from build123d import *
from build123d.topology import SkipClean

# Parameters (mm, degrees)
IZIM1_R                     = 6.5
Y_KSEKLIK_EKSTR_ZYON2_DEPTH = 15
IZIM2_R                     = 30
Y_KSEKLIK_EKSTR_ZYON3_DEPTH = 20
IZIM3_R                     = 20
KES_EKSTR_ZYON2_DEPTH       = 83
IZIM4_R                     = 2.5
KES_EKSTR_ZYON3_DEPTH       = 15


with BuildPart() as part:
    # Çizim1 → Yükseklik-Ekstrüzyon2 (new body)
    with BuildSketch(Plane(origin=(0, 0, 0), x_dir=(1, 0, 0), z_dir=(0, 1, 0))):
        with BuildLine():
            Line((-49.8, 17.348198754), (-8, 28.91366459))
            ThreePointArc((-8, 28.91366459), (0, 30), (8, 28.91366459))
            Line((8, 28.91366459), (49.8, 17.348198754))
            ThreePointArc((49.8, 17.348198754), (63, 0), (49.8, -17.348198754))
            Line((49.8, -17.348198754), (8, -28.91366459))
            ThreePointArc((8, -28.91366459), (0, -30), (-8, -28.91366459))
            Line((-8, -28.91366459), (-49.8, -17.348198754))
            ThreePointArc((-49.8, -17.348198754), (-63, 0), (-49.8, 17.348198754))
        make_face()
        with Locations(Location((-45, 0, 0), (0, 0, 270))):
            Circle(IZIM1_R, mode=Mode.SUBTRACT)
        with Locations(Location((45, 0, 0), (0, 0, 90))):
            Circle(IZIM1_R, mode=Mode.SUBTRACT)
    extrude(amount=Y_KSEKLIK_EKSTR_ZYON2_DEPTH)

    # Çizim2 → Yükseklik-Ekstrüzyon3 (add)
    with SkipClean():  # the faces are left unmerged after this step: merging them gives an invalid solid
        with BuildSketch(Plane(origin=(0, 15, 0), x_dir=(1, 0, 0), z_dir=(0, 1, 0))):
            with Locations(Location((0, 0, 0), (0, 0, 105.466009953))):
                Circle(IZIM2_R)
        extrude(amount=Y_KSEKLIK_EKSTR_ZYON3_DEPTH)

    # Çizim3 → Kes-Ekstrüzyon2 (cut)
    with SkipClean():  # the faces are left unmerged after this step: merging them gives an invalid solid
        with BuildSketch(Plane(origin=(0, 35, 0), x_dir=(1, 0, 0), z_dir=(0, 1, 0))):
            with Locations(Location((0, 0, 0), (0, 0, 270))):
                Circle(IZIM3_R)
        extrude(amount=-KES_EKSTR_ZYON2_DEPTH, mode=Mode.SUBTRACT)

    # Çizim4 → Kes-Ekstrüzyon3 (cut)
    with BuildSketch(Plane(origin=(0, 0, -30), x_dir=(-1, 0, 0), z_dir=(0, 0, -1))):
        with Locations((0, 20)):
            Circle(IZIM4_R)
    extrude(amount=-KES_EKSTR_ZYON3_DEPTH, mode=Mode.SUBTRACT)


solid = part.part
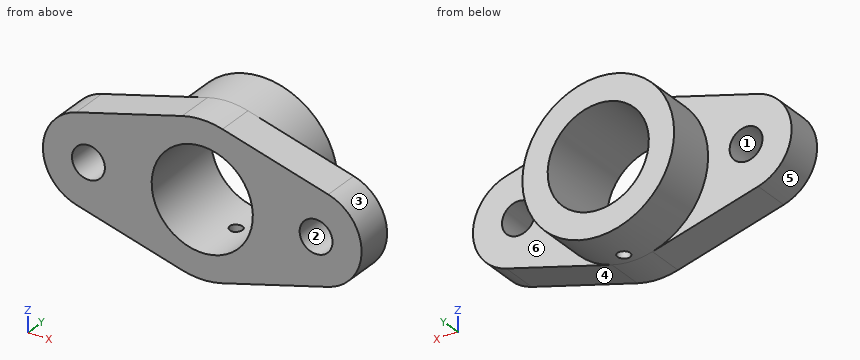
CAD build for the part. Positions are in the model's coordinates, mm. Face numbers are marked on the shaded views. A direction names the side the tool comes from. Give positions to 0.01 mm unless a question says otherwise; leave off trailing zeros. Write each loop counter-clockwise with the first axis right and the second up, starting at its lowest first coordinate (ties: lowest second). Pieces come first, ordered by that corner, then holes. Notation, with made-up numbers: (75.25, 35) -> (130.25, 35) arc R29 cw to (130.25, 55) -> close; hole circle Ø9 at (17, -29). An arc over 180 degrees is marked (long way). Return JSON: item names as keys, results as strings.
Item 1: Tool access for the marked faces 5 and 6: list every direction of +Z, -Z, +X, -X, +Y, -Y with a clear straight run to the whole face (end or side of a thin tool).
Answer below:
{"face 5": "-X, +Y, -Y", "face 6": "+X, +Y"}
Item 2: Drill centre lines: probe 1 along X at (y, z) = (10, 0); probe 2 along Z at (x, y) = (0, 25); probe 3 along Y at (x, z) = (-53.5, -7.5). Where is each one in solid material? Low to high.
Answer below:
{"probe 1": "x = -63 to -51.5, -38.5 to -20, 20 to 38.5, 51.5 to 63", "probe 2": "z = -30 to -20, 20 to 30", "probe 3": "y = 0 to 15"}
Item 3: Band-saw the part on C-C (x = 0). List the corners of the cut face in (y, z), then the cut area to 3 significant figures.
Answer below:
{"outline": "(0, -30) -> (17.5, -30) -> (17.5, -20) -> (0, -20) -> close; (0, 20) -> (35, 20) -> (35, 30) -> (0, 30) -> close; (22.5, -30) -> (35, -30) -> (35, -20) -> (22.5, -20) -> close", "area": "650 mm2"}
Item 4: Drop flat-ended pins along their axis: pin 1 (3 mm diameter, centred on x = 36, z = -8, fed in from +Y); pin 2 (2 mm diameter, centred on x = -32.5, y = 11.5, fed in from +Z); pin 3 (1 mm diameter, centred on y = 6, z = -4.5, fed in from +X). Give the stop position or say it passes through.
Answer below:
{"pin 1": "stops at y = 15", "pin 2": "stops at z = 22.41", "pin 3": "stops at x = 62.55"}
Item 5: Band-saw the part on B-B (y = 13.5). List the corners of the cut face in (x, z).
Answer below:
{"outline": "(-49.8, -17.35) -> (-8, -28.91) arc R30 ccw to (8, -28.91) -> (49.8, -17.35) arc R18 ccw to (49.8, 17.35) -> (8, 28.91) arc R30 ccw to (-8, 28.91) -> (-49.8, 17.35) arc R18 ccw to start; hole circle Ø13 at (-45, 0); hole circle Ø40 at (0, 0); hole circle Ø13 at (45, 0)"}
Item 6: Band-saw the part on A-A (z = 0). List the corners of the cut face in (x, y).
Answer below:
{"outline": "(-63, 0) -> (-51.5, 0) -> (-51.5, 15) -> (-63, 15) -> close; (-38.5, 0) -> (-20, 0) -> (-20, 35) -> (-30, 35) -> (-30, 15) -> (-38.5, 15) -> close; (20, 0) -> (38.5, 0) -> (38.5, 15) -> (30, 15) -> (30, 35) -> (20, 35) -> close; (51.5, 0) -> (63, 0) -> (63, 15) -> (51.5, 15) -> close"}
Item 7: Band-saw the part on D-D (z = 18.5). List the corners of the cut face in (x, y), then the cut area to 3 significant figures.
Answer below:
{"outline": "(-45.64, 0) -> (-7.6, 0) -> (-7.6, 35) -> (-23.62, 35) -> (-23.62, 15) -> (-45.64, 15) -> close; (7.6, 0) -> (45.64, 0) -> (45.64, 15) -> (23.62, 15) -> (23.62, 35) -> (7.6, 35) -> close", "area": "1,780 mm2"}
Item 8: Two-plate mould, pull along Z, no slides. Class the marked faces 1, 2, 3 and 4: +Z half, -Z half, draft (parallel to the pull), parting line (faces both ways), or undercut.
Answer below:
{"face 1": "undercut", "face 2": "undercut", "face 3": "parting line", "face 4": "-Z half"}
